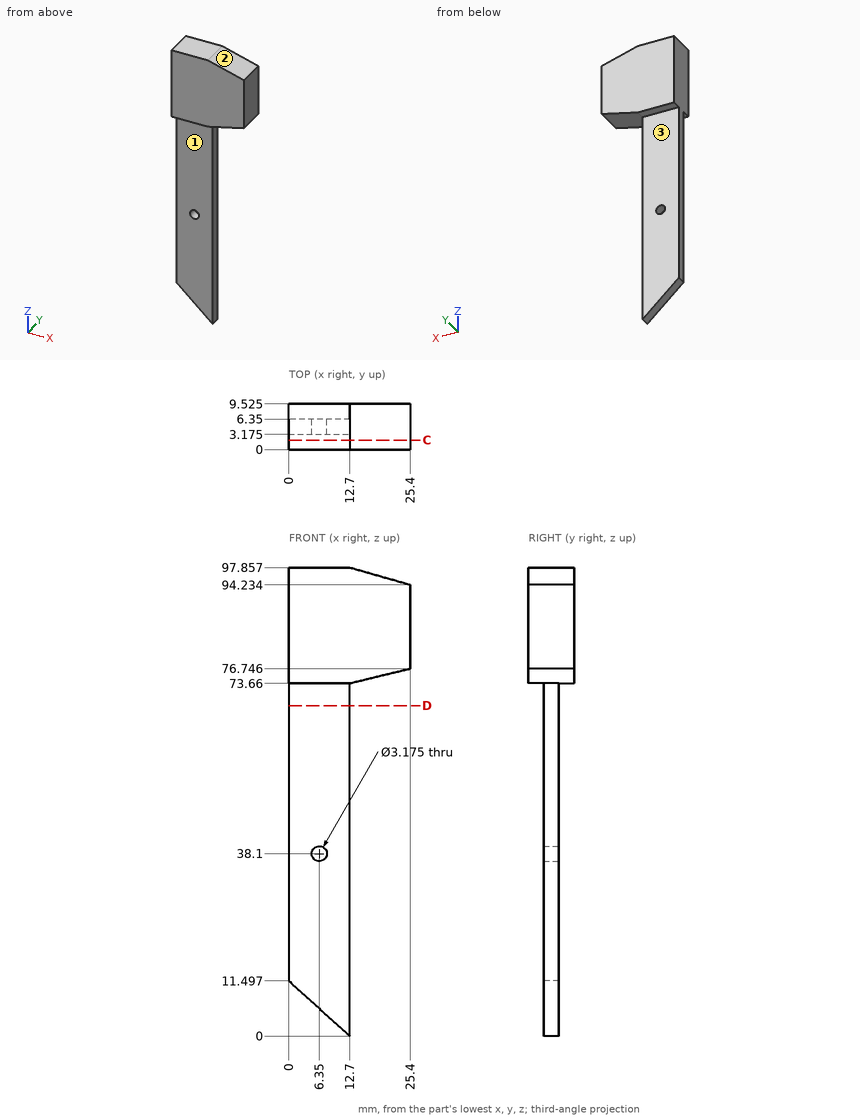
Answer from the drawing. Dimensions are ordinates in mm from the lowest x, y and z of the part. A direction names the side the tool comes from. Coordinates: 2 decimals unless noted, no trailing zeros. Order: outer loops, then holes, each group sorted by start corner. A loop starts at its lowest first (then second) coordinate and runs counter-clockwise, first axis right, second up. Notation, with made-up numbers: (-30.75, 14) - (19.25, 14) arc R15 ccw to (19.25, 28) - close; hole circle Ø1 at (16.5, 68.25). An arc over 180 degrees is marked (long way). Use one line per item in the form item = value.
(1) Which of the six approach directions +Z, -Z, +X, -X, +Y, -Y give full straight-line access (tool end or side, diameter ignored) to the marked faces 1, 2 and 3?
Computed values:
face_1 = -Z, +X, -X, -Y
face_2 = +Z, +X, +Y, -Y
face_3 = -Z, +X, -X, +Y
(2) Section C-C, the plane y = 2 is taken. Give the vertices of the cut face in (x, z), then the cut area to 3 significant figures.
Computed values:
outline = (0, 73.66) - (12.7, 73.66) - (25.4, 76.75) - (25.4, 94.23) - (12.7, 97.86) - (0, 97.86) - close
area = 572 mm²
(3) Straight lines are drawn through the part: L1, parallel to Z at x = 1, y = 8; L2, parallel to Z at x = 6.35, y = 4.95; L3, parallel to Y at x = 12.25, z = 5 (3 decimals). For each, find the intervals that lie inside material, in ascending order.
Computed values:
L1 = 73.66 to 97.86
L2 = 5.75 to 36.51, 39.69 to 97.86
L3 = 3.175 to 6.35
(4) Given pin 1 Ø3.5 at (y, z) = (5.5, 23.5) entering from +X; pin 2 Ø1 at (x, y) = (15.5, 8) entering from -Z; pin 3 Ø1 at (x, y) = (7, 8.5) entering from -Z, each flat-ended and moving along its own axis, determine where each tip first touches the part or whether it passes through.
Computed values:
pin_1 = 12.7
pin_2 = 74.22
pin_3 = 73.66
(5) Section D-D, the plane z = 69 is taken. Give the vertices of the cut face in (x, y) (3 decimals).
Computed values:
outline = (0, 3.175) - (12.7, 3.175) - (12.7, 6.35) - (0, 6.35) - close
